```python
from build123d import *

# Parameters (mm, degrees)
F0_W     = 14
F0_H     = 3
F0_W_2   = 3
F1_DEPTH = 20
F2_DEPTH = 3
F3_W     = 3
F3_H     = 3
F4_DEPTH = 100
F5_W     = 3
F5_H     = 3.5
F6_DEPTH = 100
F7_R     = 1.5
F9_DEPTH = 1


with BuildPart() as f1:
    # F0 (on Front) → F1 (new body)
    with BuildSketch(Plane.XZ):
        Polygon((10, 1.5), (10, 4.5), (-10, 4.5), (-10, 1.5), (-7, 1.5), (7, 1.5), align=None)
        Rectangle(F0_W, F0_H)
        with Locations((11.5, 0)):
            Rectangle(F0_W_2, F0_H)
        with Locations((8.5, 0)):
            Rectangle(F0_W_2, F0_H)
        with Locations((-8.5, 0)):
            Rectangle(F0_W_2, F0_H)
        Polygon((10, -4.5), (10, -1.5), (7, -1.5), (-7, -1.5), (-10, -1.5), (-10, -4.5), align=None)
    extrude(amount=-F1_DEPTH)

    # F0 (on Front) → F2 (join)
    with BuildSketch(Plane.XZ):
        with Locations((-8.5, 0)):
            Rectangle(F0_W_2, F0_H)
        Rectangle(F0_W, F0_H)
        with Locations((8.5, 0)):
            Rectangle(F0_W_2, F0_H)
        with Locations((11.5, 0)):
            Rectangle(F0_W_2, F0_H)
    extrude(amount=F2_DEPTH)

    # F3 (on face) → F4 (cut)
    with BuildSketch(Plane.YZ.offset(13)):
        Polygon((23, -1.75), (23, 1.75), (17, 1.75), (17, 1.5), (20, 1.5), (20, -1.5), (17, -1.5), (17, -1.75), align=None)
        with Locations((18.5, 0)):
            Rectangle(F3_W, F3_H)
    extrude(amount=-F4_DEPTH, mode=Mode.SUBTRACT)

    # F5 (on face) → F6 (cut)
    with BuildSketch(Plane(origin=(0, 17, 0), x_dir=(-1, 0, 0), z_dir=(0, 1, 0))):
        with Locations((11.5, 0)):
            Rectangle(F5_W, F5_H)
        with Locations((8.5, 0)):
            Rectangle(F5_W, F5_H)
    extrude(amount=-F6_DEPTH, mode=Mode.SUBTRACT)

    # F7
    f7_edges = [f1.edges().sort_by_distance(p)[0] for p in [
        (-7, -3, 0),
        (13, -3, 0),
        (10, 0, 3),
        (10, 0, -3),
        (-10, 0, -3.125),
        (-10, 0, 3.125),
        (-7, 17, 0),
        (-10, 20, 3.125),
        (-10, 20, -3.125),
        (13, 17, 0),
        (10, 20, 3.125),
        (10, 20, -3.125),
    ]]
    fillet(f7_edges, radius=F7_R)

    # F8 (on face) → F9 (cut)
    with BuildSketch(Plane.XY.offset(4.5)):
        with BuildLine():
            Line((3.824145146, 3), (7.4031382015, 3))
            Line((7.4031382015, 3), (4.5441972293, 5.7829861111))
            add(Edge.make_bspline(
                [(5.902270146, 7.9416232639), (5.3037458404, 6.7217881944), (4.5441972293, 5.7829861111)],
                knots=[0, 0, 0, 1, 1, 1], degree=2))
            add(Edge.make_bspline(
                [(6.8441104237, 10.4435763889), (6.5007944515, 9.1614583333), (5.902270146, 7.9416232639)],
                knots=[0, 0, 0, 1, 1, 1], degree=2))
            Line((6.8441104237, 10.4435763889), (3.824145146, 10.4435763889))
            add(Edge.make_bspline(
                [(2.6574784793, 7.5846354167), (3.3289194515, 8.6966145833), (3.824145146, 10.4435763889)],
                knots=[0, 0, 0, 1, 1, 1], degree=2))
            Line((2.6574784793, 7.5846354167), (-0.0404381874, 10.2157118056))
            add(Edge.make_bspline(
                [(2.0771833404, 11.99609375), (1.4209333404, 11.0603298611), (-0.0404381874, 10.2157118056)],
                knots=[0, 0, 0, 1, 1, 1], degree=2))
            add(Edge.make_bspline(
                [(2.7334333404, 14.0620659722), (2.7334333404, 12.9318576389), (2.0771833404, 11.99609375)],
                knots=[0, 0, 0, 1, 1, 1], degree=2))
            add(Edge.make_bspline(
                [(1.6746225765, 16.2586805556), (2.7334333404, 15.4383680556), (2.7334333404, 14.0620659722)],
                knots=[0, 0, 0, 1, 1, 1], degree=2))
            add(Edge.make_bspline(
                [(-1.152417354, 17.0789930556), (0.6158118126, 17.0789930556), (1.6746225765, 16.2586805556)],
                knots=[0, 0, 0, 1, 1, 1], degree=2))
            add(Edge.make_bspline(
                [(-4.1085805485, 16.1963975694), (-3.0026777707, 17.0789930556), (-1.152417354, 17.0789930556)],
                knots=[0, 0, 0, 1, 1, 1], degree=2))
            add(Edge.make_bspline(
                [(-5.2144833263, 13.8706597222), (-5.2144833263, 15.3138020833), (-4.1085805485, 16.1963975694)],
                knots=[0, 0, 0, 1, 1, 1], degree=2))
            add(Edge.make_bspline(
                [(-4.8924347151, 12.2437065972), (-5.2144833263, 12.9895833333), (-5.2144833263, 13.8706597222)],
                knots=[0, 0, 0, 1, 1, 1], degree=2))
            add(Edge.make_bspline(
                [(-3.8564104096, 10.6805555556), (-4.570386104, 11.4978298611), (-4.8924347151, 12.2437065972)],
                knots=[0, 0, 0, 1, 1, 1], degree=2))
            add(Edge.make_bspline(
                [(-5.828198604, 8.9685329861), (-5.253979854, 9.8845486111), (-3.8564104096, 10.6805555556)],
                knots=[0, 0, 0, 1, 1, 1], degree=2))
            add(Edge.make_bspline(
                [(-6.402417354, 6.7491319444), (-6.402417354, 8.0525173611), (-5.828198604, 8.9685329861)],
                knots=[0, 0, 0, 1, 1, 1], degree=2))
            add(Edge.make_bspline(
                [(-5.0443444374, 3.8734809028), (-6.402417354, 4.9383680556), (-6.402417354, 6.7491319444)],
                knots=[0, 0, 0, 1, 1, 1], degree=2))
            add(Edge.make_bspline(
                [(-3.1611686995, 3), (-4.2620419441, 3.260064742), (-5.0443444374, 3.8734809028)],
                knots=[0.4239613473, 0.4239613473, 0.4239613473, 1, 1, 1], degree=2))
            Line((-3.1611686995, 3), (0.3406843845, 3))
            add(Edge.make_bspline(
                [(2.7334333404, 4.0724826389), (1.6254830234, 3.300443557), (0.3406843845, 3)],
                knots=[0, 0, 0, 0.6108441088, 0.6108441088, 0.6108441088], degree=2))
            Line((2.7334333404, 4.0724826389), (3.824145146, 3))
        make_face()
        with BuildLine():
            add(Edge.make_bspline(
                [(-3.3551083263, 7.0256076389), (-3.3551083263, 6.2083333333), (-2.7413930485, 5.7252604167)],
                knots=[0, 0, 0, 1, 1, 1], degree=2))
            add(Edge.make_bspline(
                [(-3.0360979096, 8.0798611111), (-3.3551083263, 7.6241319444), (-3.3551083263, 7.0256076389)],
                knots=[0, 0, 0, 1, 1, 1], degree=2))
            add(Edge.make_bspline(
                [(-2.1671742985, 8.9518229167), (-2.7170874929, 8.5355902778), (-3.0360979096, 8.0798611111)],
                knots=[0, 0, 0, 1, 1, 1], degree=2))
            Line((-2.1671742985, 8.9518229167), (0.9864715349, 5.8194444444))
            add(Edge.make_bspline(
                [(-1.1706465207, 5.2421875), (0.0264020904, 5.2421875), (0.9864715349, 5.8194444444)],
                knots=[0, 0, 0, 1, 1, 1], degree=2))
            add(Edge.make_bspline(
                [(-2.7413930485, 5.7252604167), (-2.1276777707, 5.2421875), (-1.1706465207, 5.2421875)],
                knots=[0, 0, 0, 1, 1, 1], degree=2))
        make_face(mode=Mode.SUBTRACT)
        with BuildLine():
            add(Edge.make_bspline(
                [(0.0537458404, 13.7582465278), (0.0537458404, 14.2595486111), (-0.2880510346, 14.5496961806)],
                knots=[0, 0, 0, 1, 1, 1], degree=2))
            add(Edge.make_bspline(
                [(-0.3822350624, 12.7267795139), (0.0537458404, 13.1688368056), (0.0537458404, 13.7582465278)],
                knots=[0, 0, 0, 1, 1, 1], degree=2))
            add(Edge.make_bspline(
                [(-1.6354902707, 11.8289930556), (-0.8182159651, 12.2847222222), (-0.3822350624, 12.7267795139)],
                knots=[0, 0, 0, 1, 1, 1], degree=2))
            add(Edge.make_bspline(
                [(-2.5378340207, 13.6731770833), (-2.5378340207, 12.8376736111), (-1.6354902707, 11.8289930556)],
                knots=[0, 0, 0, 1, 1, 1], degree=2))
            add(Edge.make_bspline(
                [(-2.1717315901, 14.5360243056), (-2.5378340207, 14.2322048611), (-2.5378340207, 13.6731770833)],
                knots=[0, 0, 0, 1, 1, 1], degree=2))
            add(Edge.make_bspline(
                [(-1.1706465207, 14.83984375), (-1.8056291596, 14.83984375), (-2.1717315901, 14.5360243056)],
                knots=[0, 0, 0, 1, 1, 1], degree=2))
            add(Edge.make_bspline(
                [(-0.2880510346, 14.5496961806), (-0.6298479096, 14.83984375), (-1.1706465207, 14.83984375)],
                knots=[0, 0, 0, 1, 1, 1], degree=2))
        make_face(mode=Mode.SUBTRACT)
    extrude(amount=-F9_DEPTH, mode=Mode.SUBTRACT)


solid = f1.part
```
Input: part model. Units: mm. Frame: model coordinates. A direction names the side the tool comes from. Round coordinates to 2 decimals unless told otherwise and drop trailing zeros. Write each loop counter-clockwise with the first axis right and the second up, starting at its lowest first coordinate (ties: lowest second). Pieces come first, ordered by that corner, then holes. Notation, with made-up numbers: (-25, -30.75) -> (31, -30.75) arc R14 cw to (31, -17.75) -> close; hole circle Ø9 at (73.25, -20.5). An arc over 180 degrees is marked (long way). Answer as CSV lines item,"result".
1. Ray query, L1, parallel to Z at x = -7.25, y = 9.5; L2, parallel to X at y = 14, z = 2.5; L3, parallel to Y at x = -4.25, z = 4. Return the intervals inside material, ascending. Write a range as [from, to].
Geometry says:
L1,"z = [-4.5, -1.75], [1.75, 4.5]"
L2,"x = [-10, 10]"
L3,"y = [0, 3.38], [10.44, 11.17], [16.08, 20]"
2. Mould query, pull axis X, two halves, no side actions, for faces 1 (the cylindrical face through (-9.57, 19.55, 3.11)), 2 (the cylindrical face through (12.55, -2.57, 0.02)), 3 (the flat face through (-1, 3, 4)), 4 (the flat face through (3, -3, 0)). Classes: +X half, -X half, draft (parallel to the pull), parting line (faces both ways), or undercut.
Geometry says:
face 1,"-X half"
face 2,"+X half"
face 3,"undercut"
face 4,"draft"
3. Reachability of faces 5 (the flat face through (3, 17, 0)), 6 (the flat face through (-1, 9, 3.5)), 7 (the flat face through (5.9, -0.4, -1.5)) from +Z, -Z, +X, -X, +Y, -Y: full face, straight path, thin tool, end or side. Return the list, or none.
Geometry says:
face 5,"+X, -X, +Y"
face 6,"+Z"
face 7,"-Z, +X, -Y"
4. Section B-B (y = 1). Return the cut outline in (x, z), plus the area to 3 significant figures.
Geometry says:
outline,"(-9.91, -4.5) -> (9.91, -4.5) -> (9.91, -1.5) -> (13, -1.5) -> (13, 1.5) -> (9.91, 1.5) -> (9.91, 4.5) -> (-9.91, 4.5) -> (-9.91, 1.75) -> (-7, 1.75) -> (-7, -1.75) -> (-9.91, -1.75) -> close"
area,"178 mm^2"
5. Contact query for flat-ended pins moving along their axis: P1, Ø1, axis at x = 6, z = 0.5, coming from the +Y side; P2, Ø2.5, axis at y = 14, z = 3.5, coming from the +X side; P3, Ø1.8, axis at y = 3.5, z = 0, coming from the -X side. Output: stop coordinate, or through.
Geometry says:
P1,"stops at y = 17"
P2,"stops at x = 10"
P3,"stops at x = -7"
6. Section A-A (z = 1). Return the cut outline in (x, y).
Geometry says:
outline,"(-7, -1.5) arc R1.5 ccw to (-5.5, -3) -> (11.5, -3) arc R1.5 ccw to (13, -1.5) -> (13, 15.5) arc R1.5 ccw to (11.5, 17) -> (-5.5, 17) arc R1.5 ccw to (-7, 15.5) -> close"
7. Section C-C (x = 10.75). Return the cut outline in (y, z).
Geometry says:
outline,"(-3, -1.5) -> (17, -1.5) -> (17, 1.5) -> (-3, 1.5) -> close"
